from build123d import *

# Parameters (mm, degrees)
EXTRUDE_1_DEPTH = 18
M20X2_5_1_D     = 32
M20X2_5_1_DEPTH = 47.5
M20X2_5_1_TIP   = 9.613769904


with BuildPart() as part:
    # 草图1 → 拉伸1 (new body)
    with BuildSketch(Plane.XY):
        Polygon((26.558112383, 0), (13.279056191, 23), (-13.279056191, 23), (-26.558112383, 0), (-13.279056191, -23), (13.279056191, -23), align=None)
    extrude(amount=EXTRUDE_1_DEPTH)

    # 草图2 → 切除-旋转1 (revolve, cut)
    with BuildSketch(Plane(origin=(0, 0, 0), x_dir=(1, 0, 0), z_dir=(0, 1, 0))):
        Polygon((4.209845782, 9.902777738), (26.558112383, -3), (32.141291251, 6.670349468), align=None)
        Polygon((26.558112383, -15), (32.141291251, -24.670349468), (4.209845782, -27.902777738), align=None)
    revolve(axis=Axis((0, 0, -13.306273389), (0, 0, 1)), mode=Mode.SUBTRACT)

    # M20x2.5 螺纹孔1
    with Locations(Plane.XY.offset(18)):
        with Locations((0, 0)):
            Hole(M20X2_5_1_D / 2, depth=M20X2_5_1_DEPTH)
            with Locations((0, 0, -(M20X2_5_1_DEPTH + M20X2_5_1_TIP / 2))):  # 118° drill point
                Cone(0, M20X2_5_1_D / 2, M20X2_5_1_TIP, mode=Mode.SUBTRACT)


solid = part.part
Source: CAD feature listing. Evaluate the final solid. Frame: model axes, mm. Give positions to 0.01 mm unless a question says otherwise; leave off trailing zeros. Order: outer loops, then holes, each group sorted by start corner. A loop starts at its lowest first (then second) coordinate and runs counter-clockwise, first axis right, second up. Notation, with made-up numbers: (-38.5, -13.75) -> (16.5, -13.75) arc R13 ccw to (16.5, -2.75) -> close; hole circle Ø11 at (2.5, 37.25). An arc over 180 degrees is marked (long way). Use a Markdown table: item, result.
1) Section query B-B, the plane x = 0. Return the cut outline in (y, z).
Answer list:
| item | result |
|---|---|
| outline | (-23, 0.95) -> (-21.36, 0) -> (-16, 0) -> (-16, 18) -> (-21.36, 18) -> (-23, 17.05) -> close; (16, 0) -> (21.36, 0) -> (23, 0.95) -> (23, 17.05) -> (21.36, 18) -> (16, 18) -> close |
2) Contact query for flat-ended pins moving along their axis: P1, Ø2, axis at x = 5, y = 17.5, coming from the -Z side; P2, Ø12, axis at x = 5.5, y = 2.5, coming from the +Z side; P3, Ø10, axis at y = 9, z = 15, coming from the -X side; P4, Ø3, axis at y = 5.5, z = 7.5, coming from the +X side. Output: stop coordinate, or through.
Answer list:
| item | result |
|---|---|
| P1 | z = 0 |
| P2 | through |
| P3 | x = -24.25 |
| P4 | x = 24.25 |
3) Ray query, line 1 along Y through (x, z) = (0, 8.5); line 2 along Z through (x, y) = (-4, 21); line 3 along Y through (x, z) = (9.5, 4.5). Return the intervals inside material, ascending. Write a range as [from, to].
Answer list:
| item | result |
|---|---|
| line 1 | [-23, -16], [16, 23] |
| line 2 | [0.01, 17.99] |
| line 3 | [-23, -12.87], [12.87, 23] |
4) Section query A-A, the plane z = 4.5. Return the cut outline in (x, y), then the cut area to 3 significant figures.
Answer list:
| item | result |
|---|---|
| outline | (-26.56, 0) -> (-13.28, -23) -> (13.28, -23) -> (26.56, 0) -> (13.28, 23) -> (-13.28, 23) -> close; hole circle Ø32 at (0, 0) |
| area | 1,030 mm² |
5) Mould query, pull axis Y, two halves, no side actions, for faces 1 (the cylindrical face through (3.47, -15.62, 8.87)), 2 (the flat face through (3, 16, 0)), 3 (the flat face through (20.01, 11.34, 8.89)). Classes: +Y half, -Y half, draft (parallel to the pull), parting line (faces both ways), or undercut.
Answer list:
| item | result |
|---|---|
| face 1 | undercut |
| face 2 | draft |
| face 3 | +Y half |
